Check sheet for the drawn part. Datum: minimum x, y, z corner. Units: mm. A direction names the side the tool comes from. Coordinates: 2 decimals unless noted, no trailing zeros. Loops run counter-clockwise (first coordinate to the right, second up) from the corner with the lowest first, then second, coordinate; pieces in that order, holes last. Notation, with made-up numbers: (58.25, -6.5) - (115.25, -6.5) arc R30 cw to (115.25, 25.5) - close; hole circle Ø7 at (61.5, -23.75). An arc over 180 degrees is marked (long way). Write item = value, one per line. Start each with the question number.
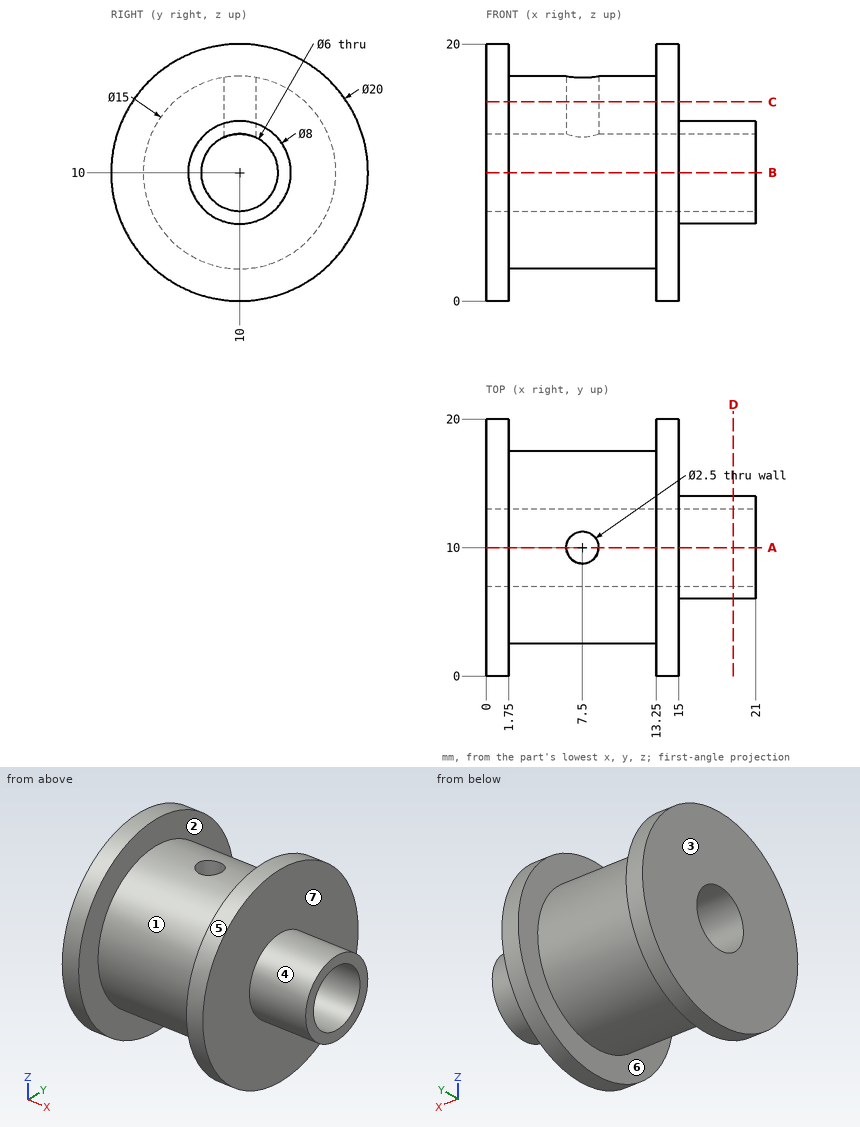
(1) Depth check by flat-ended pin: pin 1 (10 mm diameter, centred on x = 13.5, y = 10.5, fed in from -Z); pin 2 (4 mm diameter, centred on x = 19, y = 10, fed in from +Z); pin 3 (5 mm diameter, centred on x = 7, y = 8.5, fed in from +Z); pin 4 (1.5 mm diameter, centred on x = 7.5, y = 10, fed in from +Z). Enter the tip coordinate at first touch or a pass-through.
(2) Draft check along X on the marked faces 1, 2, 3 and 4. Enter one of: pulls with the +X half, pulls with the -X half, needs draft (parallel to the pull), parting line crosses it, or undercut.
(3) Tool access check on the marked faces 5, 6 and 7. Record the directions out of +Z, -Z, +X, -X, +Y, -Y that give a thin tool (end or side, any length) a straight path to the whole face; none if there is none.
(4) Sectioned sample at B-B on z = 10. Enter the section's corners in (x, y).
(5) Sectioned sample at A-A on y = 10. Enter the section's corners in (x, z).
(6) Sectioned sample at D-D on x = 19.25. Enter the section's corners in (y, z).
(7) Scan lines: line 1 (X direction, y = 16.25, z = 5.5); line 2 (Y direction, x = 11.25, z = 10); line 3 (X direction, y = 10, z = 13.95). Record each from-to range of solid material in increasing order.
(8) Sectioned sample at C-C on z = 15.5. Enter the section's corners in (x, y).
Working result:
q1.pin_1 = 0
q1.pin_2 = 14
q1.pin_3 = 17.5
q1.pin_4 = 7.1
q2.face_1 = undercut
q2.face_2 = undercut
q2.face_3 = pulls with the -X half
q2.face_4 = needs draft
q3.face_5 = +X, -X
q3.face_6 = none
q3.face_7 = +X
q4.outline = (0, 0) - (1.75, 0) - (1.75, 2.5) - (13.25, 2.5) - (13.25, 0) - (15, 0) - (15, 6) - (21, 6) - (21, 7) - (0, 7) - close; (0, 13) - (21, 13) - (21, 14) - (15, 14) - (15, 20) - (13.25, 20) - (13.25, 17.5) - (1.75, 17.5) - (1.75, 20) - (0, 20) - close
q5.outline = (0, 0) - (1.75, 0) - (1.75, 2.5) - (13.25, 2.5) - (13.25, 0) - (15, 0) - (15, 6) - (21, 6) - (21, 7) - (0, 7) - close; (0, 13) - (6.25, 13) - (6.25, 17.5) - (1.75, 17.5) - (1.75, 20) - (0, 20) - close; (8.75, 13) - (21, 13) - (21, 14) - (15, 14) - (15, 20) - (13.25, 20) - (13.25, 17.5) - (8.75, 17.5) - close
q6.outline = circle Ø8 at (10, 10); hole circle Ø6 at (10, 10)
q7.line_1 = 0 to 1.75, 13.25 to 15
q7.line_2 = 2.5 to 7, 13 to 17.5
q7.line_3 = 0 to 6.25, 8.75 to 21
q8.outline = (0, 1.65) - (1.75, 1.65) - (1.75, 4.9) - (13.25, 4.9) - (13.25, 1.65) - (15, 1.65) - (15, 18.35) - (13.25, 18.35) - (13.25, 15.1) - (1.75, 15.1) - (1.75, 18.35) - (0, 18.35) - close; hole circle Ø2.5 at (7.5, 10)
